Design review of the part built by this model. Coordinates are the model's own, in mm. A direction names the side the tool comes from. Give positions to 0.01 mm unless a question says otherwise; leave off trailing zeros. Order: outer loops, then holes, each group sorted by start corner. A loop starts at its lowest first (then second) coordinate and runs counter-clockwise, first axis right, second up. Notation, with made-up numbers: M 2,-4 L 36,-4 A15 cw 36,22 Z; hole C 88.25,60 d9. An arc over 180 degrees is marked long. Answer as a JSON object with one key per item and string values.
from build123d import *

# Parameters (mm, degrees)
SKETCH_1_W             = 30
SKETCH_1_H             = 15
EXTRUDE_1_DEPTH        = 40
EXTRUDE_2_DEPTH        = 5
SKETCH_3_R             = 3
CUT_EXTRUDE_1_DEPTH    = 5
EXTRUDE_3_DEPTH        = 7.5
SKETCH_7_R             = 3
EXTRUDE_4_DEPTH        = 7
EXTRUDE_5_DEPTH        = 5
FILLET_2_R             = 1.5
FILLET_3_R             = 0.5
FILLET_3_OF_MIRROR_3_R = 0.5


with BuildPart() as part:
    # 草图1 → 凸台-拉伸1 (new body)
    with BuildSketch(Plane.XY):
        Rectangle(SKETCH_1_W, SKETCH_1_H)
    extrude(amount=EXTRUDE_1_DEPTH)

    # 草图2 → 凸台-拉伸2 (add)
    with BuildSketch(Plane(origin=(15, 0, 0), x_dir=(0, 0, -1), z_dir=(1, 0, 0))):
        with BuildLine():
            Line((-40, -7.5), (-48, -7.5))
            ThreePointArc((-48, -7.5), (-55.5, 0), (-48, 7.5))
            Line((-48, 7.5), (-40, 7.5))
            Line((-40, 7.5), (-40, -7.5))
        make_face()
    extrude_2 = extrude(amount=-EXTRUDE_2_DEPTH)

    # 草图3 → 切除-拉伸1 (cut)
    with BuildSketch(Plane(origin=(15, 0, 0), x_dir=(0, 0, -1), z_dir=(1, 0, 0))):
        with Locations(Location((-48, 0, 0), (0, 0, 90))):
            Circle(SKETCH_3_R)
    cut_extrude_1 = extrude(amount=-CUT_EXTRUDE_1_DEPTH, mode=Mode.SUBTRACT)

    # 镜向1: 凸台-拉伸2, 切除-拉伸1 across plane
    add(extrude_2.mirror(Plane(origin=(0, 0, 0), x_dir=(0, 0, 1), z_dir=(1, 0, 0))))
    add(cut_extrude_1.mirror(Plane(origin=(0, 0, 0), x_dir=(0, 0, 1), z_dir=(1, 0, 0))), mode=Mode.SUBTRACT)

    # 草图6 → 凸台-拉伸3 (add, symmetric)
    with BuildSketch(Plane(origin=(0, 0, 0), x_dir=(0, 0, -1), z_dir=(1, 0, 0))):
        with BuildLine():
            Line((0, 7.5), (8, 7.5))
            ThreePointArc((8, 7.5), (15.5, 0), (8, -7.5))
            Line((8, -7.5), (0, -7.5))
            Line((0, -7.5), (0, 7.5))
        make_face()
    extrude(amount=EXTRUDE_3_DEPTH, both=True)

    # 草图7 → 凸台-拉伸4 (add)
    with BuildSketch(Plane(origin=(7.5, 0, 0), x_dir=(0, 0, -1), z_dir=(1, 0, 0))):
        with Locations(Location((8, 0, 0), (0, 0, 180))):
            Circle(SKETCH_7_R)
    extrude_4 = extrude(amount=EXTRUDE_4_DEPTH)

    # 镜向2: 凸台-拉伸4 across plane
    add(extrude_4.mirror(Plane(origin=(0, 0, 0), x_dir=(0, 0, 1), z_dir=(1, 0, 0))))

    # 草图8 → 凸台-拉伸5 (add)
    with BuildSketch(Plane(origin=(15, 0, 0), x_dir=(0, 0, -1), z_dir=(1, 0, 0))):
        with BuildLine():
            Line((-56.810546127, 10.5), (-52.820907073, 5.745333323))
            ThreePointArc((-52.820907073, 5.745333323), (-50.565151075, 7.047694656), (-48, 7.5))
            Line((-48, 7.5), (-44.01973259, 7.5))
            Line((-44.01973259, 7.5), (-44.01973259, 10.5))
            Line((-44.01973259, 10.5), (-56.810546127, 10.5))
        make_face()
    extrude_5 = extrude(amount=-EXTRUDE_5_DEPTH)

    # 圆角2
    fillet_2_edges = [part.edges().sort_by_distance(p)[0] for p in [
        (12.5, 7.5, 44.01973259),
    ]]
    fillet(fillet_2_edges, radius=FILLET_2_R)
    fillet_2_2_edges = [part.edges().sort_by_distance(p)[0] for p in [
        (12.5, 10.5, 44.01973259),
    ]]
    fillet(fillet_2_2_edges, radius=FILLET_2_R - 0.0001)  # a hair under: the kernel refuses the full size

    # 圆角3
    fillet_3_edges = [part.edges().sort_by_distance(p)[0] for p in [
        (12.5, 10.5, 56.810546127),
    ]]
    fillet(fillet_3_edges, radius=FILLET_3_R)

    # 镜向3: 凸台-拉伸5 across plane
    add(extrude_5.mirror(Plane(origin=(0, 0, 0), x_dir=(0, 0, 1), z_dir=(1, 0, 0))))

    # 圆角3 of 镜向3
    fillet_3_of_mirror_3_edges = [part.edges().sort_by_distance(p)[0] for p in [
        (-12.5, 10.5, 56.810546127),
    ]]
    fillet(fillet_3_of_mirror_3_edges, radius=FILLET_3_OF_MIRROR_3_R)


solid = part.part
(1) Insertion check: pin 1 (5.5 mm diameter, centred on y = 0, z = 48, fed in from -X); pin 2 (1.8 mm diameter, centred on y = 0, z = -9, fed in from +X); pin 3 (2 mm diameter, centred on x = -1.5, z = 18.5, fed in from +Y); pin 4 (3 mm diameter, centred on y = -0.5, z = -9, fed in from -X). Each pin has a flat end and moves straight along its axis. Give the tip position at first contact, or say it passes through.
Checked values:
{"pin 1": "passes through", "pin 2": "stops at x = 14.5", "pin 3": "stops at y = 7.5", "pin 4": "stops at x = -14.5"}
(2) Tool access review of faces 1 (the flat face through (14.5, 0, -8)), 2 (the cylindrical face through (10.95, 1.15, -5.23)), 3 (the cylindrical face through (12.5, 10, 44.4)): name each direction out of +Z, -Z, +X, -X, +Y, -Y from which nothing blocks a thin tool from reaching the whole face with its end or side.
Checked values:
{"face 1": "-Z, +X, +Y, -Y", "face 2": "+X", "face 3": "-Z, +X, +Y"}
(3) Draft analysis for pull direction X (two halves, no side actions). For faces 4 (the flat face through (10, 4, 48)), 5 (the flat face through (15, 0, 29)), 6 (the cylindrical face through (-10.95, 1.15, -5.23)), state which applies: +X half, -X half, draft (parallel to the pull), parting line (faces both ways), or undercut.
Checked values:
{"face 4": "undercut", "face 5": "+X half", "face 6": "draft"}
(4) We need section A-A (x = 12.75). Count the separate pieces of the cut face and the enclosed holes in it, plus the area to 3 significant figures.
Checked values:
{"separate pieces": "2", "enclosed holes": "1", "area": "847 mm^2"}
(5) We need section D-D (z = 3.5). Write out the cut boundary in (x, y), plus the area to 3 significant figures.
Checked values:
{"outline": "M -15,-7.5 L 15,-7.5 L 15,7.5 L -15,7.5 Z", "area": "450 mm^2"}
(6) We need section C-C (x = 9.25). Write out the cut boundary in (y, z), plus the area to 3 significant figures.
Checked values:
{"outline": "M -7.5,0 L 7.5,0 L 7.5,40 L -7.5,40 Z; C 0,-8 d6", "area": "628 mm^2"}
(7) To check wall thickness, follow L1, parallel to X at y = 5, z = 46.5; L2, parallel to X at y = 5.75, z = -1.5. State the ranges of each line that lie inside material, in increasing order. Write a range as from..to.
Checked values:
{"L1": "x = -15..-10, 10..15", "L2": "x = -7.5..7.5"}
(8) We need section B-B (y = 0). Write out the cut boundary in (x, z), plus the area to 3 significant figures.
Checked values:
{"outline": "M -15,0 L -7.5,0 L -7.5,-5 L -14.5,-5 L -14.5,-11 L -7.5,-11 L -7.5,-15.5 L 7.5,-15.5 L 7.5,-11 L 14.5,-11 L 14.5,-5 L 7.5,-5 L 7.5,0 L 15,0 L 15,45 L 10,45 L 10,40 L -10,40 L -10,45 L -15,45 Z; M -15,51 L -10,51 L -10,55.5 L -15,55.5 Z; M 10,51 L 15,51 L 15,55.5 L 10,55.5 Z", "area": "1,610 mm^2"}
